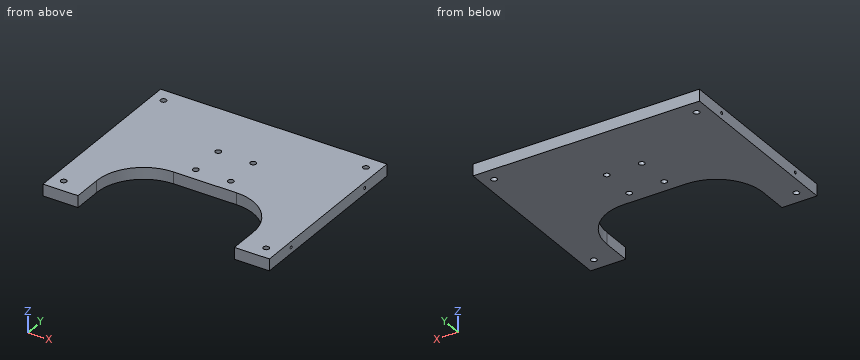
from build123d import *

# Parameters (mm, degrees)
BOSS_EXTRUDE1_DEPTH         = 12.7
F_1_4_0_25_DIAMETER_HOLE1_D = 6.35
FILLET2_R                   = 50.8
HOLE1_AT_2_COUNT            = 2
HOLE1_AT_2_PITCH            = 125.108514383


with BuildPart() as part:
    # Sketch1 → Boss-Extrude1 (new body)
    with BuildSketch(Plane.XY):
        Polygon((258.933482757, 10.713854335), (12.7, 10.713854335), (12.7, -189.051843155), (50.8, -189.051843155), (50.8, -106.501843155), (220.833482757, -106.501843155), (220.833482757, -189.051843155), (258.933482757, -189.051843155), align=None)
    extrude(amount=-BOSS_EXTRUDE1_DEPTH)

    # 1/4 (0.25) Diameter Hole1 (through all)
    with Locations(Plane(origin=(0, 0, -12.7), x_dir=(-1, 0, 0), z_dir=(0, 0, -1))):
        with Locations((-25.706162889, -174.233423282), (-116.766741379, -92.064314729), (-154.866741379, -92.064314729), (-245.927319868, -174.233423282), (-154.866741379, -53.964314729), (-245.927319868, -4.747970506), (-116.766741379, -53.964314729), (-25.706162889, -4.747970506)):
            Hole(F_1_4_0_25_DIAMETER_HOLE1_D / 2)

    # Fillet2
    fillet2_edges = [part.edges().sort_by_distance(p)[0] for p in [
        (220.833482757, -106.501843155, -6.35),
        (50.8, -106.501843155, -6.35),
    ]]
    fillet(fillet2_edges, radius=FILLET2_R)

    # Sketch7 → Hole1 (revolve, cut)
    with BuildSketch(Plane(origin=(0, -152.193459623, -6.35), x_dir=(0, 0, 1), z_dir=(0, 1, 0))):
        Polygon((0, 0), (0, 39.053866233), (1.5875, 38.1), (1.5875, 4.017661662), (5.08, 0), align=None)
    hole1 = revolve(axis=Axis((-14.308894879, -152.193459623, -6.35), (1, 0, 0)), mode=Mode.SUBTRACT)

    # Hole1 at 2: Hole1 ×2
    with Locations(*[(0, i * HOLE1_AT_2_PITCH, 0) for i in range(1, HOLE1_AT_2_COUNT)]):
        add(hole1, mode=Mode.SUBTRACT)

    # Mirror1: Hole1 across plane
    add(hole1.mirror(Plane.ZY.offset(-135.816741379)), mode=Mode.SUBTRACT)

    # Mirror1 copy 1 sketch → Mirror1 copy 1 (revolve, cut)
    with BuildSketch(Plane(origin=(271.633482757, -27.08494524, -6.35), x_dir=(0, 0, 1), z_dir=(0, 1, 0))):
        Polygon((0, 0), (0, -39.053866233), (1.5875, -38.1), (1.5875, -4.017661662), (5.08, 0), align=None)
    revolve(axis=Axis((285.942377636, -27.08494524, -6.35), (1, 0, 0)), mode=Mode.SUBTRACT)


solid = part.part
The listing builds one solid part. Answer for the finished solid, in the listing's coordinates (mm). Coordinates: 2 decimals unless noted, no trailing zeros. Write each loop counter-clockwise with the first axis right and the second up, starting at its lowest first coordinate (ties: lowest second). Pieces come first, ordered by that corner, then holes. Notation, with made-up numbers: (57, 61) - (96, 61) arc R29 ccw to (96, 94) - close; hole circle Ø6 at (69, 62.5). An arc over 180 degrees is marked (long way). Answer as CSV lines item,"result".
1. Straight lines are drawn through the part: line 1 (X direction, y = -92.5, z = -5); line 2 (Y direction, x = 241.75, z = -6.35); line 3 (Y direction, x = 26, z = -4.5). For each, find the intervals that lie inside material, in ascending order. Write a range as [from, to].
Computed values:
line 1,"x = [12.7, 113.62], [119.91, 151.72], [158.01, 258.93]"
line 2,"y = [-189.05, -153.78], [-150.61, -28.67], [-25.5, 10.71]"
line 3,"y = [-189.05, -177.39], [-171.07, -7.91], [-1.59, 10.71]"
2. Find section A-A (y = -143). Give the vertices of the cut face in (x, z).
Computed values:
outline,"(12.7, -12.7) - (52.85, -12.7) - (52.85, 0) - (12.7, 0) - close; (218.78, -12.7) - (258.93, -12.7) - (258.93, 0) - (218.78, 0) - close"
3. Find section D-D (x = 177.5). Give the vertices of the cut face in (y, z).
Computed values:
outline,"(-107.05, -12.7) - (10.71, -12.7) - (10.71, 0) - (-107.05, 0) - close"
4. Given P1, Ø3, axis at y = -27.08, z = -6.35, coming from the +X side, flat-ended and moving along its own axis, determine where the tip first touches the part or whether it passes through.
Computed values:
P1,"stops at x = 233.48"
5. Find section C-C (x = 136.5). Give the vertices of the cut face in (y, z), plus the area to 3 significant figures.
Computed values:
outline,"(-106.5, -12.7) - (10.71, -12.7) - (10.71, 0) - (-106.5, 0) - close"
area,"1,490 mm²"
6. Find section B-B (z = -2). Give the number of separate pieces and of enclosed holes in the cut face, plus the area to 3 significant figures.
Computed values:
separate pieces,"1"
enclosed holes,"8"
area,"36,000 mm²"
